Part model, mm, in its own coordinate system. A direction names the side the tool comes from. Coordinates: 2 decimals unless noted, no trailing zeros. Loops run counter-clockwise (first coordinate to the right, second up) from the corner with the lowest first, then second, coordinate; pieces in that order, holes last. Notation, with made-up numbers: (85, 19.25) -> (94, 19.25) arc R10 ccw to (94, 32.25) -> close; hole circle Ø8 at (32, -21.75). An arc over 180 degrees is marked (long way). One line per item, written item: value. Start each with the question number.
from build123d import *

# Parameters (mm, degrees)
F0_W     = 41.147999
F0_H     = 41.605201
F1_DEPTH = 5.08
F2_W     = 11.5824
F2_H     = 41.605201
F3_DEPTH = 34.544
F4_W     = 29.565599
F4_H     = 14.0208
F5_DEPTH = 14.224
F7_D     = 13.462


with BuildPart() as f1:
    # F0 (on Top) → F1 (new body)
    with BuildSketch(Plane.XY):
        with Locations((-20.573999, 20.802601)):
            Rectangle(F0_W, F0_H)
    extrude(amount=F1_DEPTH)

    # F2 (on face) → F3 (join)
    with BuildSketch(Plane.XY.offset(5.08)):
        with Locations((-5.7912, 20.802601)):
            Rectangle(F2_W, F2_H)
    extrude(amount=F3_DEPTH)

    # F4 (on face) → F5 (join)
    with BuildSketch(Plane.XY.offset(5.08)):
        with Locations((-26.365199, 20.4216)):
            Rectangle(F4_W, F4_H)
    extrude(amount=F5_DEPTH)

    # F7 (through all)
    with Locations(Plane(origin=(-41.147999, 0, 0), x_dir=(0, -1, 0), z_dir=(-1, 0, 0))):
        with Locations((-20.4216, 19.304)):
            Hole(F7_D / 2)


solid = f1.part
1) Pin check, flat tips, straight feed: pin 1 Ø7 at (x, y) = (-24, 32.5) entering from +Z; pin 2 Ø7 at (x, z) = (-20.5, 15) entering from -Y; pin 3 Ø2 at (y, z) = (30, 30) entering from -X. Stop position of each tip, or through.
2) Probe line 1 (X direction, y = 14.5, z = 32.5); line 2 (Y direction, x = -12, z = 16.5); line 3 (Z direction, x = -19, y = 39). List the from-to ranges inside material, lowest first. Write a range as from..to.
3) Slice it at A-A (x = -25). Give the cut face in (y, z), then the cut area to 3 significant figures.
4) Slice it at D-D (z = 10). Give the cut face in (x, y).
5) Pull direction Y, two halves, no side cores. Call faces 1 (the cylindrical face through (-15.714, 23.528, 13.332)), 2 (the flat face through (-21, 21, 0)), 3 (the flat face through (-27, 27.432, 12)): +Y half, -Y half, draft (parallel to the pull), parting line (faces both ways), or undercut.
6) Slice it at C-C (y = 8). Give the cut face in (x, z).
7) Slice it at B-B (y = 20.5). Give the cut face in (x, z).
8) Tool access for faces 4 (the flat face through (-10, 0, 14)), 5 (the flat face through (-27, 35, 5.08)), 6 (the flat face through (-27, 13.411, 12)): list every direction of +Z, -Z, +X, -X, +Y, -Y with a clear straight run to the whole face (end or side of a thin tool).
Check sheet entries:
1. pin 1: stops at z = 5.08
1. pin 2: stops at y = 13.41
1. pin 3: stops at x = -11.58
2. line 1: x = -11.58..0
2. line 2: y = 13.41..14.3, 26.54..27.43
2. line 3: z = 0..5.08
3. outline: (0, 0) -> (41.61, 0) -> (41.61, 5.08) -> (27.43, 5.08) -> (27.43, 19.3) -> (27.15, 19.3) arc R6.73 cw to (13.69, 19.3) -> (13.41, 19.3) -> (13.41, 5.08) -> (0, 5.08) -> close
3. area: 340 mm^2
4. outline: (-41.15, 13.41) -> (-11.58, 13.41) -> (-11.58, 0) -> (0, 0) -> (0, 41.61) -> (-11.58, 41.61) -> (-11.58, 27.43) -> (-41.15, 27.43) -> close
5. face 1: undercut
5. face 2: draft
5. face 3: +Y half
6. outline: (-41.15, 0) -> (0, 0) -> (0, 39.62) -> (-11.58, 39.62) -> (-11.58, 5.08) -> (-41.15, 5.08) -> close
7. outline: (-41.15, 0) -> (0, 0) -> (0, 12.57) -> (-41.15, 12.57) -> close; (-11.58, 26.03) -> (0, 26.03) -> (0, 39.62) -> (-11.58, 39.62) -> close
8. face 4: +Z, -Z, +X, -X, -Y
8. face 5: +Z, -X, +Y
8. face 6: +Z, -X, -Y
